Design review of the part shown in the three views and the two pictorial views. Dimensions are in mm from the part's minimum x, y and z. A direction names the side the tool comes from. Round coordinates to 2 decimals unless told otherwise and drop trailing zeros. Loops run counter-clockwise (first coordinate to the right, second up) from the corner with the lowest first, then second, coordinate; pieces in that order, holes last.
1. Consider section A-A on y = 4.5. State the section outline as (x, z) points.
2. Consider section C-C on x = 22.5. State the section outline as (y, z) points.
3. Consider section B-B on x = 12. State the section outline as (y, z) points.
4. Tool access review of the marked faces 1 and 2: name each direction out of +Z, -Z, +X, -X, +Y, -Y from which nothing blocks a thin tool from reaching the whole face with its end or side.
5. Clearance check with flat-ended pins moving along their axes: pin 1 Ø4 at (x, z) = (17.5, 4) entering from -Y; pin 2 Ø10 at (x, z) = (14.5, 8) entering from +Y; pin 3 Ø5 at (x, z) = (10.5, 17) entering from +Y; pin 4 Ø1.5 at (y, z) = (2, 17) entering from +X. State where each tip first meets the part, or that it passes through.
6. Draft analysis for pull direction X (two halves, no side actions). For the marked faces 3, 4, 5 and 6, state which applies: released by +X, released by -X, zero draft, split by the parting line, or undercut.
7. To check wall thickness, follow line 1 along Z through (x, y) = (12, 8.25); line 2 along Z through (x, y) = (11.75, 6.25). State the ranges of each line that lie inside material, in increasing order.
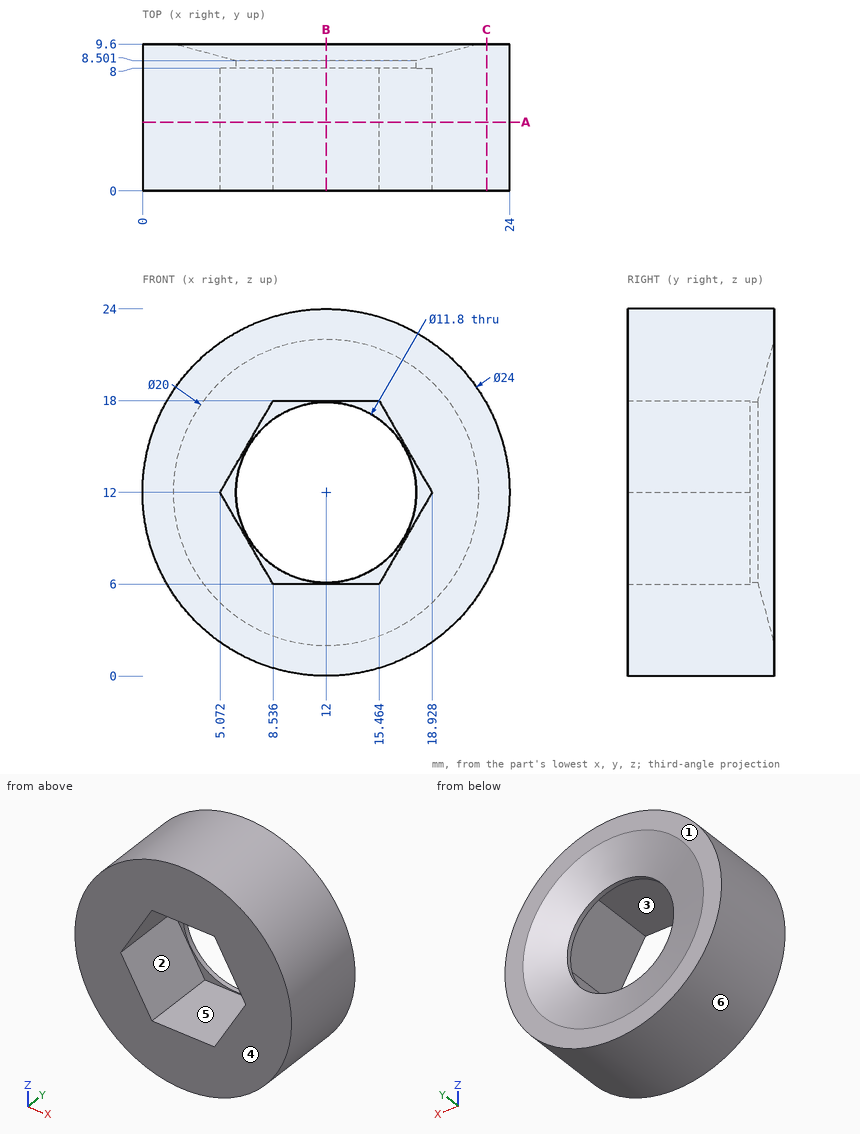
Resolved:
1. outline: circle Ø24 at (12, 12); hole (5.07, 12) - (8.54, 6) - (15.46, 6) - (18.93, 12) - (15.46, 18) - (8.54, 18) - close
2. outline: (0, 6.19) - (9.6, 6.19) - (9.6, 17.81) - (0, 17.81) - close
3. outline: (0, 0) - (9.6, 0) - (9.6, 2) - (8.5, 6.1) - (8, 6.1) - (8, 6) - (0, 6) - close; (0, 18) - (8, 18) - (8, 17.9) - (8.5, 17.9) - (9.6, 22) - (9.6, 24) - (0, 24) - close
4. face 1: +Z, -Z, +X, -X, +Y
4. face 2: -Y
5. pin 1: stops at y = 0
5. pin 2: stops at y = 9.52
5. pin 3: stops at y = 8.99
5. pin 4: stops at x = 23.22
6. face 3: undercut
6. face 4: zero draft
6. face 5: undercut
6. face 6: split by the parting line
7. line 1: z = 0 to 6.1, 17.9 to 24
7. line 2: z = 0 to 6, 18 to 24
